Geometry check sheet. Reference: drawing and pictorial views, mm from the part's lowest x, y, z. A direction names the side the tool comes from. Give positions to 0.01 mm unless a question says otherwise; leave off trailing zeros. Answer as a JSON object with one key per item and string values. Group by question number.
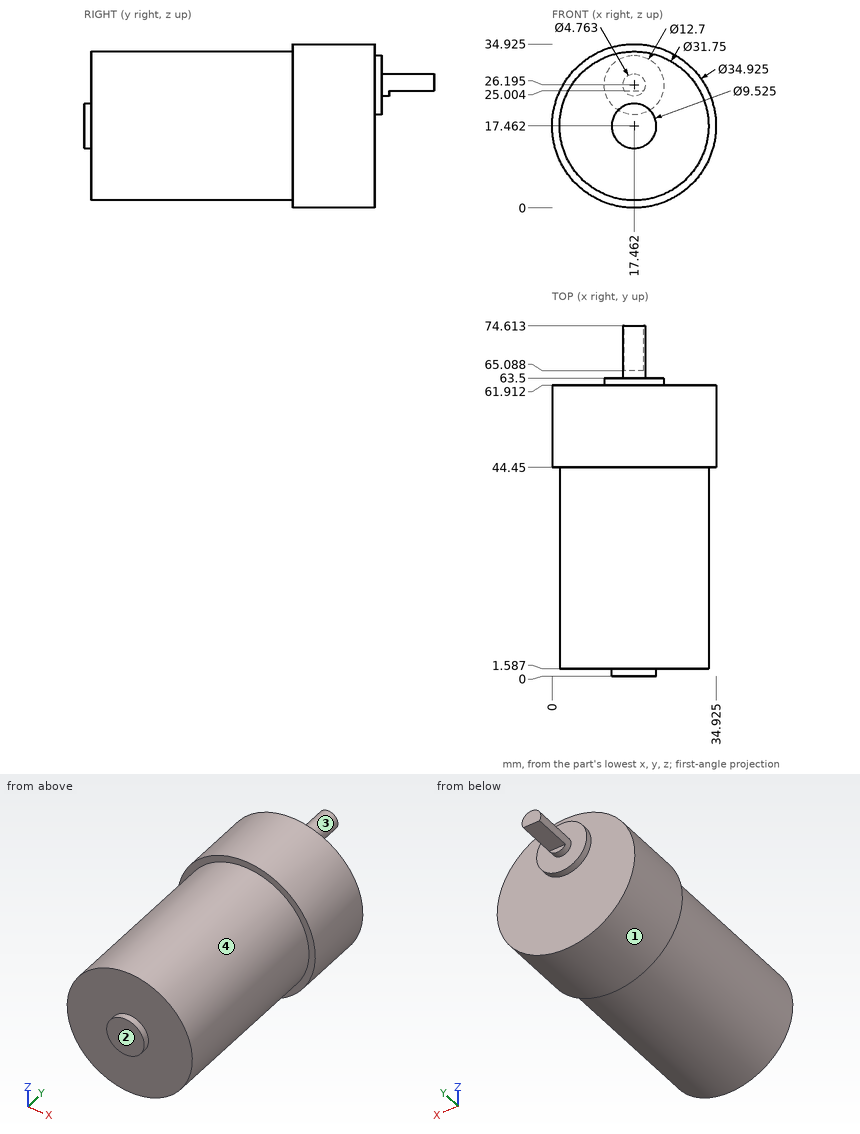
1. Release check for a two-part mould opening along Z. For the marked faces 1 and 2 record: released by +Z, released by -Z, zero draft, split by the parting line, or undercut.
2. Thickness scan on line 1 along Y through (x, z) = (33, 11.5); line 2 along X through (y, z) = (13, 18); line 3 along Y through (x, z) = (13, 2.5). Record the ranges inside material, lowest first. Write a range as [from, to].
3. Depth check by flat-ended pin: pin 1 (3 mm diameter, centred on x = 16, z = 30, fed in from -Y); pin 2 (1.5 mm diameter, centred on x = 21, y = 18.5, fed in from -Z); pin 3 (3 mm diameter, centred on y = 28, z = 29.5, fed in from +X) (1 decimal); pin 4 (6 mm diameter, centred on x = 9, y = 67, fed in from +Z). Enter the tip coordinate at first touch or a pass-through.
4. Access from +Z, -Z, +X, -X, +Y, -Y to the whole of each face (thin tool, end or side, straight path). Record for the marked faces 3 and 4.
Report:
{
 "1": {"face 1": "split by the parting line", "face 2": "zero draft"},
 "2": {"line 1": "y = [44.45, 61.91]", "line 2": "x = [1.6, 33.33]", "line 3": "y = [1.59, 61.91]"},
 "3": {"pin 1": "stops at y = 1.59", "pin 2": "stops at z = 1.83", "pin 3": "stops at x = 29.3", "pin 4": "passes through"},
 "4": {"face 3": "+Y", "face 4": "-Y"}
}
